```python
from build123d import *

# Parameters (mm, degrees)
F1_DEPTH = 38.1
F2_R     = 12.7
F3_DEPTH = 533.4
F4_W     = 127
F4_H     = 38.1
F5_DEPTH = 25.4


with BuildPart() as f1:
    # F0 (on Top) → F1 (new body)
    with BuildSketch(Plane.XY):
        Polygon((-46.300181, 91.77144), (-71.700181, 91.77144), (-71.700181, -35.22856), (-46.300181, -35.22856), (-46.300181, 15.57144), (-46.300181, 40.97144), align=None)
    extrude(amount=F1_DEPTH)

    # F2 (on face) → F3 (join)
    with BuildSketch(Plane.YZ.offset(-46.300181)):
        with Locations((28.27144, 19.05)):
            Circle(F2_R)
    extrude(amount=F3_DEPTH)

    # F4 (on face) → F5 (join)
    with BuildSketch(Plane.YZ.offset(487.099819)):
        with Locations((28.27144, 19.05)):
            Rectangle(F4_W, F4_H)
    extrude(amount=F5_DEPTH)


solid = f1.part
```
The listing builds one solid part. Answer for the finished solid, in the listing's coordinates (mm). A direction names the side the tool comes from. Round coordinates to 2 decimals unless told otherwise and drop trailing zeros. Order: outer loops, then holes, each group sorted by start corner. A loop starts at its lowest first (then second) coordinate and runs counter-clockwise, first axis right, second up. Notation, with made-up numbers: (-20.75, 30.5) - (27.25, 30.5) arc R16 cw to (27.25, 61.5) - close; hole circle Ø10 at (-12, 29.5). An arc over 180 degrees is marked (long way). Put each result on its own line as item: value. Start each with the question number.
(1) Determine the mould class of faces 1 (the flat face through (-59, -35.229, 19)), 2 (the flat face through (487.1, 27, 32)), 3 (the flat face through (512.5, 27, 19)) for opening direction X: released by +X, released by -X, zero draft, split by the parting line, or undercut.
(2) Find section C-C (y = 23). Give the vertices of the cut face in (x, z).
(3) Find section D-D (x = 334). Give the vertices of the cut face in (y, z).
(4) Given P1, Ø3, axis at x = 192.5, z = 16.5, coming from the -Y side; P2, Ø5, axis at x = 247.5, z = 10, coming from the -Y side; P3, Ø1, axis at x = 7.5, z = 26, coming from the +Y side, each flat-ended and moving along its own axis, determine where each tip first touches the part or whether it passes through.
(5) Find section B-B (z = 19.05). Give the vertices of the cut face in (x, y), plus the area to 3 significant figures.
(6) For faces 4 (the cylindrical face through (216.67, 25.52, 6.65)), 5 (the flat face through (-59, 29, 38.1)), determine the directions among +Z, -Z, +X, -X, +Y, -Y from which every point of the face is accessible in a straight line to the end or side of a thin tool.
(7) Straight lines are drawn through the part: probe 1 along X at (y, z) = (2.5, 25); probe 2 along Z at (x, y) = (470.5, 28.5); probe 3 along Y at (x, z) = (118, 19). For each, find the intervals that lie inside material, in ascending order. Write a range as from..to.
(8) Find section A-A (y = -13.5). Give the vertices of the cut face in (x, z).
Reply:
1. face 1: zero draft
1. face 2: undercut
1. face 3: released by +X
2. outline: (-71.7, 0) - (-46.3, 0) - (-46.3, 7.5) - (487.1, 7.5) - (487.1, 0) - (512.5, 0) - (512.5, 38.1) - (487.1, 38.1) - (487.1, 30.6) - (-46.3, 30.6) - (-46.3, 38.1) - (-71.7, 38.1) - close
3. outline: circle Ø25.4 at (28.27, 19.05)
4. P1: y = 15.61
4. P2: y = 17.39
4. P3: y = 39.21
5. outline: (-71.7, -35.23) - (-46.3, -35.23) - (-46.3, 15.57) - (487.1, 15.57) - (487.1, -35.23) - (512.5, -35.23) - (512.5, 91.77) - (487.1, 91.77) - (487.1, 40.97) - (-46.3, 40.97) - (-46.3, 91.77) - (-71.7, 91.77) - close
5. area: 20,000 mm^2
6. face 4: none
6. face 5: +Z, +X, -X, +Y, -Y
7. probe 1: -71.7..-46.3, 487.1..512.5
7. probe 2: 6.35..31.75
7. probe 3: 15.57..40.97
8. outline: (-71.7, 0) - (-46.3, 0) - (-46.3, 38.1) - (-71.7, 38.1) - close; (487.1, 0) - (512.5, 0) - (512.5, 38.1) - (487.1, 38.1) - close
